Source: CAD feature listing. Evaluate the final solid. Frame: model axes, mm. Give positions to 0.01 mm unless a question says otherwise; leave off trailing zeros. Write each loop counter-clockwise with the first axis right and the second up, starting at its lowest first coordinate (ties: lowest second). Pieces come first, ordered by that corner, then holes. Notation, with made-up numbers: M -34.75,38 L -27.75,38 A16 cw -27.75,68 Z; hole C 2,3.5 d9. An arc over 180 degrees is marked long. Use CSV: the item, a comma, the result in double quotes. Start each with the question number.
from build123d import *

# Parameters (mm, degrees)
REVOLVE1_ANGLE = 360


with BuildPart() as part:
    # Sketch2 → Revolve1 (revolve, symmetric)
    with BuildSketch(Plane.XY) as revolve1_sk:
        Polygon((-393.7, 0), (-393.7, 3.175), (-379.4125, 3.175), (-379.4125, 5.715), (-375.840625, 5.715), (-375.840625, 16.775092336), (-374.65, 17.4625), (374.65, 17.4625), (375.840625, 16.775092336), (375.840625, 5.715), (379.4125, 5.715), (379.4125, 3.175), (393.7, 3.175), (393.7, 0), align=None)
    revolve(axis=Axis((-393.7, 0, 0), (1, 0, 0)), revolution_arc=REVOLVE1_ANGLE / 2)
    revolve(revolve1_sk.sketch, axis=Axis((-393.7, 0, 0), (-1, 0, 0)), revolution_arc=REVOLVE1_ANGLE / 2)


solid = part.part
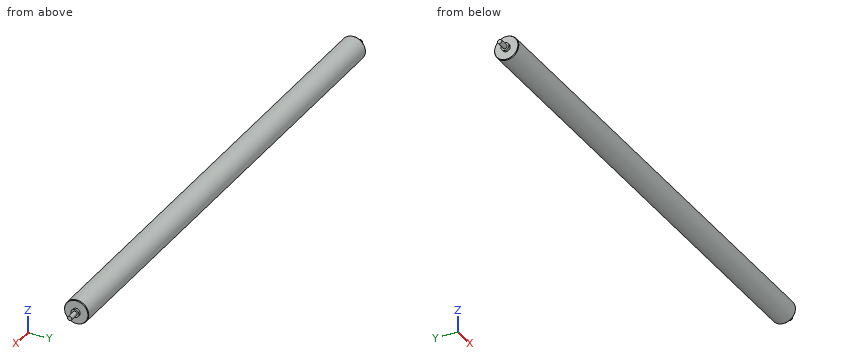
Item 1: Section A-A (x = -257). Return the cut outline in (y, z) (1 decimal).
Item 2: Material intervals for probe 1 along X at (y, z) = (-8, -6.5); probe 2 along Y at (x, z) = (-306, 0.5); probe 3 along Z at (x, y) = (-238, -4.5), sorted ascending.
Item 3: Contact query for flat-ended pins moving along their axis: pin 1 Ø10 at (y, z) = (12, -3) entering from +X; pin 2 Ø1 at (y, z) = (-13, -10.5) entering from -X; pin 3 Ø5 at (y, z) = (1.5, 7) entering from -X. Output: stop coordinate, or through.
Output values:
1,outline,"C 0,0 d34.9"
2,probe 1,"x = -375.84 to 375.84"
2,probe 2,"y = -17.46 to 17.46"
2,probe 3,"z = -16.87 to 16.87"
3,pin 1,"stops at x = 375.84"
3,pin 2,"stops at x = -375.84"
3,pin 3,"stops at x = -379.41"
